CAD build for the part. Positions are in the model's coordinates, mm. A direction names the side the tool comes from. Coordinates: 2 decimals unless noted, no trailing zeros. Order: outer loops, then holes, each group sorted by start corner. A loop starts at its lowest first (then second) coordinate and runs counter-clockwise, first axis right, second up. Notation, with made-up numbers: M 89,39.5 L 94,39.5 A15 cw 94,50.5 Z; hole C 21.5,59.5 d2. An arc over 180 degrees is marked long. Write item = value, one per line. Start each with the question number.
Autodesk Inventor part; units mm, degrees
ref_plane "Work Plane1" through (0, 0, 40) normal (0, 0, 1) x (1, 0, 0)
ref_plane "YZ Plane" through (0, 0, 0) normal (1, 0, 0) x (0, 1, 0)
ref_plane "XZ Plane" through (0, 0, 0) normal (0, 1, 0) x (-1, 0, 0)
sketch "Sketch1" plane through (0, 0, 0) normal (0, 0, 1) x (1, 0, 0)
  line L0 (17, 5) -> (17, -3.2)
  line L1 (17, -3.2) -> (12, -3.2)
  line L2 (12, -12.5) -> (12, -9)
  line L3 (12, -9) -> (17, -9)
  line L4 (17, -9) -> (17, -17.5)
  line L5 (17, -17.5) -> (0, -17.5)
  line L6 (0, -17.5) -> (0, 0)
  line L7 (17, 5) -> (-6, 5)
  line L8 (-6, 5) -> (-6, 0)
  line L9 (-6, 0) -> (0, 0)
  line L10 (12, -3.2) -> (12, 0.3)
  line L11 (12, -12.5) -> (8, -12.5)
  line L12 (8, -12.5) -> (8, 0.3)
  line L13 (8, 0.3) -> (12, 0.3)
  dimension "d0" = 6
  dimension "d1" = 5
  dimension "d4" = 4
  dimension "d8" = 5
  dimension "d10" = 5.8
  dimension "d12" = 3.5
  dimension "d13" = 3.5
  dimension "d17" = 0.3
  dimension "d18" = 17
  dimension "d19" = 8
  dimension "d20" = 0
extrude "Extrusion1" add sketch "Sketch1" along normal blind 80
sketch "Sketch2" plane through (17, -17.5, 0) normal (1, 0, 0) x (0, 0, -1)
  line L0 (0, 0) -> (-80, 0)
  circle A0 centre (-24.5, 0) radius 3.5
  line L1 (0, 0) -> (0, 8.5)
  line L2 (0, 8.5) -> (-80, 8.5)
  line L3 (-80, 0) -> (-80, 8.5)
  line L4 (0, 0) -> (-80, 0)
  point P0 (0, 17.5)
  dimension "d22" = 7
  dimension "d24" = 24.5
extrude "Extrusion2" cut sketch "Sketch2" against normal blind 20 contours A0 L0 | L0 A0
ref_plane "Work Plane1" through (0, 0, 40) normal (0, 0, 1) x (1, 0, 0)
mirror "Mirror1" about plane through (0, 0, 40) normal (0, 0, 1) of "Extrusion2"
equation "\"d13\" = d12"
equation "\"d22\" = d21"
properties part number "Riel acople de motor"
1. Probe L1, parallel to X at y = -0.25, z = 64; L2, parallel to Y at x = 8.5, z = 66.5; L3, parallel to Y at x = 15.25, z = 74.5. List the from-to ranges inside material, lowest first.
2. Flat gauge pins, fed straight in: pin 1 (5 mm diameter, centred on y = -9, z = 34, fed in from -X); pin 2 (3 mm diameter, centred on x = -3.5, z = 25.5, fed in from -Y); pin 3 (2.5 mm diameter, centred on x = 15.5, z = 56.5, fed in from -Y). Where does each tip first touch, or does it go through?
3. Slice it at C-C (z = 24.5). Write the cut outline in (x, y), plus the area to 3 significant figures.
4. 3-axis set-ups, long thin cutter, end or side, ignore diameter. For faces 1 (the flat face through (15, -3.2, 39)), 2 (the flat face through (12, -11, 39)), 3 (the flat face through (0, -9, 39)): which of +Z, -Z, +X, -X, +Y, -Y reach the whole face in a straight line?
5. Mould opens along X. For faces 4 (the flat face through (12, -1, 39)), 5 (the flat face through (-6, 3, 39)), 6 (the flat face through (9, -17.5, 69)) say: released by +X, released by -X, zero draft, split by the parting line, or undercut.
6. Slice it at A-A (y = -11). Write the cut outline in (x, z), plus the area to 3 significant figures.
7. Slice it at B-B (x = 4.75). Write the cut outline in (y, z).
8. Slice it at D-D (y = -6.5). Write the cut outline in (x, z), plus the area to 3 significant figures.
Calculated:
q1.L1 = 0 to 8, 12 to 17
q1.L2 = -17.5 to -12.5, 0.3 to 5
q1.L3 = -17.5 to -9, -3.2 to 5
q2.pin_1 = 0
q2.pin_2 = 0
q2.pin_3 = -14.82
q3.outline = M -6,0 L 0,0 L 0,-14 L 17,-14 L 17,-9 L 12,-9 L 12,-12.5 L 8,-12.5 L 8,0.3 L 12,0.3 L 12,-3.2 L 17,-3.2 L 17,5 L -6,5 Z
q3.area = 273 mm²
q4.face_1 = +Z, -Z, +X
q4.face_2 = +Z, -Z
q4.face_3 = +Z, -Z, -X, -Y
q5.face_4 = undercut
q5.face_5 = released by -X
q5.face_6 = zero draft
q6.outline = M 0,0 L 8,0 L 8,80 L 0,80 Z; M 12,0 L 17,0 L 17,80 L 12,80 Z
q6.area = 1,040 mm²
q7.outline = M -17.5,0 L 5,0 L 5,80 L -17.5,80 L -17.5,59 A3.5 cw -17.5,52 L -17.5,28 A3.5 cw -17.5,21 Z
q8.outline = M 0,0 L 8,0 L 8,80 L 0,80 Z
q8.area = 640 mm²
